Read the model definition and answer for the solid it produces. Units are mm, in the model's axes. A direction names the side the tool comes from. Give positions to 0.01 mm unless a question says otherwise; leave off trailing zeros. Order: outer loops, then holes, each group sorted by start corner. A loop starts at its lowest first (then second) coordinate and runs counter-clockwise, first axis right, second up.
```python
from build123d import *

# Parameters (mm, degrees)
F1_DEPTH = 63.5
F0_W     = 25.4
F0_H     = 19.05
F2_DEPTH = 25.4
F3_DEPTH = 7.9375
F5_R     = 6.35


with BuildPart() as f1:
    # F0 (on Front) → F1 (new body, symmetric)
    with BuildSketch(Plane.XZ):
        Polygon((22.225, 9.525), (-41.275, 9.525), (-41.275, -9.525), (41.275, -9.525), (41.275, 9.525), align=None)
    extrude(amount=F1_DEPTH, both=True)

    # F0 (on Front) → F2 (join, symmetric)
    with BuildSketch(Plane.XZ):
        with BuildLine():
            Line((57.15, 45.2454016253), (60.325, 45.2454016253))
            Line((60.325, 45.2454016253), (60.325, 64.2954016253))
            Line((60.325, 64.2954016253), (57.15, 64.2954016253))
            ThreePointArc((57.15, 64.2954016253), (32.4542956671, 54.0661059583), (22.225, 29.3704016253))
            Line((22.225, 29.3704016253), (22.225, 9.525))
            Line((22.225, 9.525), (41.275, 9.525))
            Line((41.275, 9.525), (41.275, 29.3704016253))
            ThreePointArc((41.275, 29.3704016253), (45.9246798487, 40.5957217767), (57.15, 45.2454016253))
        make_face()
        with Locations((73.025, 54.7704016253)):
            Rectangle(F0_W, F0_H)
    extrude(amount=F2_DEPTH, both=True)

    # F0 (on Front) → F3 (join, symmetric)
    with BuildSketch(Plane.XZ):
        with BuildLine():
            ThreePointArc((22.225, 29.3704016253), (32.4542956671, 54.0661059583), (57.15, 64.2954016253))
            add(Edge.make_bspline(
                [(-41.275, 9.525), (-41.275, 40.0696797542), (16.9853791595, 64.2954016253), (57.15, 64.2954016253)],
                knots=[0, 0, 0, 0, 112.6378156713, 112.6378156713, 112.6378156713, 112.6378156713], degree=3))
            Line((-41.275, 9.525), (22.225, 9.525))
            Line((22.225, 9.525), (22.225, 29.3704016253))
        make_face()
    extrude(amount=F3_DEPTH, both=True)

    # F0 (on Front) → F4 (revolve)
    with BuildSketch(Plane.XZ):
        Polygon((85.725, 45.2454016253), (85.725, 38.1), (111.125, 38.1), (111.125, 66.675), (85.725, 66.675), (85.725, 64.2954016253), align=None)
    revolve(axis=Axis((85.725, 0, 52.3875), (0, 0, 1)))

    # F5
    f5_edges = [f1.edges().sort_by_distance(p)[0] for p in [
        (-41.275, -63.5, 0),
        (41.275, -63.5, 0),
        (41.275, 63.5, 0),
        (-41.275, 63.5, 0),
    ]]
    fillet(f5_edges, radius=F5_R)


solid = f1.part
```
1) Consider L1, parallel to Z at x = 88, y = -20.5 (3 decimals); L2, parallel to Z at x = 20.5, y = -31.5 (3 decimals); L3, parallel to X at y = 38, z = -1 (3 decimals). Determine where each line is inside the solid, lowest interval first.
Final values:
L1: z = 38.1 to 66.675
L2: z = -9.525 to 9.525
L3: x = -41.275 to 41.275
2) A tool of negligible diameter and unlimited length cuts with its end or side. For faces 4 (the face through (1, -36, 9.525)), 5 (the face through (60, 2, 45.245)), 6 (the face through (41.275, -1, 5)), 7 (the face through (60, -2, 64.295)), from which of +Z, -Z, +X, -X, +Y, -Y can it reach the whole face along a straight path? Write none if from no direction.
Final values:
face 4: +Z, -X, -Y
face 5: -Z
face 6: -Z, +X, +Y, -Y
face 7: +Z, -X
3) Given pin 1 (5 mm diameter, centred on y = 18.5, z = 19, fed in from -X) (3 decimals); pin 2 (5 mm diameter, centred on y = -16.5, z = 51.5, fed in from +X); pin 3 (11.5 mm diameter, centred on y = 7, z = 14, fed in from +X) (3 decimals), each flat-ended and moving along its own axis, determine where each tip first touches the part or whether it passes through.
Final values:
pin 1: stops at x = 22.225
pin 2: stops at x = 106.92
pin 3: stops at x = 41.275
4) The part is cut by section B-B on y = 39.5. Determine the outline of the cut face in (x, z) (3 decimals).
Final values:
outline: (-41.275, -9.525) - (41.275, -9.525) - (41.275, 9.525) - (-41.275, 9.525) - close
5) The part is cut by section A-A on z = 3.5. Determine the outline of the cut face in (x, y) (3 decimals), and give its area (3 significant figures).
Final values:
outline: (-41.275, -57.15) arc R6.35 ccw to (-34.925, -63.5) - (34.925, -63.5) arc R6.35 ccw to (41.275, -57.15) - (41.275, 57.15) arc R6.35 ccw to (34.925, 63.5) - (-34.925, 63.5) arc R6.35 ccw to (-41.275, 57.15) - close
area: 10,400 mm2
6) For a pull along X with two mould halves and no side action, classify faces 1 (the face through (1, 35, 9.525)), 2 (the face through (45.8, -0.36, 40.47)), 3 (the face through (22.225, -17, 20)) as released by +X, released by -X, zero draft, split by the parting line, or undercut.
Final values:
face 1: zero draft
face 2: undercut
face 3: released by -X
